For this review, take the finished solid that the model builds, in its own axes (mm). A direction names the side the tool comes from. Coordinates: 2 decimals unless noted, no trailing zeros. Loops run counter-clockwise (first coordinate to the right, second up) from the corner with the lowest first, then second, coordinate; pieces in that order, holes last. Notation, with made-up numbers: M -18.5,21.25 L 8.5,21.25 A35 cw 8.5,56.25 Z; hole C 58.5,38 d9. An arc over 180 degrees is marked long. Use one line per item in the form item = value.
```python
from build123d import *

# Parameters (mm, degrees)
SKETCH1_W           = 50
SKETCH1_H           = 50
BOSS_EXTRUDE1_DEPTH = 10
CUT_EXTRUDE3_DEPTH  = 6.3
SKETCH5_R           = 9
SKETCH5_R_2         = 3.1
BOSS_EXTRUDE2_DEPTH = 6
SKETCH6_R           = 2.7
BOSS_EXTRUDE3_DEPTH = 2.5
FILLET1_R           = 0.5
CUT_EXTRUDE4_DEPTH  = 57.789083458
FILLET2_R           = 5
CHAMFER1_SIZE       = 1
CHAMFER2_SIZE       = 1
CHAMFER2_SIZE2      = 1.414213562
FILLET3_R           = 2
SKETCH9_R           = 3.1
CUT_EXTRUDE5_DEPTH  = 37.434050008
CHAMFER3_SIZE       = 1
CUT_EXTRUDE6_DEPTH  = 6
FILLET4_R           = 3


with BuildPart() as part:
    # Sketch1 → Boss-Extrude1 (new body)
    with BuildSketch(Plane(origin=(0, 0, 0), x_dir=(1, 0, 0), z_dir=(0, 1, 0))):
        Rectangle(SKETCH1_W, SKETCH1_H)
    extrude(amount=BOSS_EXTRUDE1_DEPTH)

    # Sketch4 → Cut-Extrude3 (cut)
    with BuildSketch(Plane(origin=(0, 0, 0), x_dir=(-1, 0, 0), z_dir=(0, -1, 0))):
        with BuildLine():
            Line((21, -7.228416147), (21, -10.5))
            ThreePointArc((21, -10.5), (20.267766953, -12.267766953), (18.5, -13))
            Line((18.5, -13), (-18.5, -13))
            ThreePointArc((-18.5, -13), (-20.267766953, -12.267766953), (-21, -10.5))
            Line((-21, -10.5), (-21, -7.228416147))
            ThreePointArc((-21, -7.228416147), (-20.591644852, -6.017356006), (-19.533333333, -5.300838508))
            ThreePointArc((-19.533333333, -5.300838508), (-15.5, 0), (-19.533333333, 5.300838508))
            ThreePointArc((-19.533333333, 5.300838508), (-20.591644852, 6.017356006), (-21, 7.228416147))
            Line((-21, 7.228416147), (-21, 10.5))
            ThreePointArc((-21, 10.5), (-20.267766953, 12.267766953), (-18.5, 13))
            Line((-18.5, 13), (18.5, 13))
            ThreePointArc((18.5, 13), (20.267766953, 12.267766953), (21, 10.5))
            Line((21, 10.5), (21, 7.228416147))
            ThreePointArc((21, 7.228416147), (20.591644852, 6.017356006), (19.533333333, 5.300838508))
            ThreePointArc((19.533333333, 5.300838508), (15.5, 0), (19.533333333, -5.300838508))
            ThreePointArc((19.533333333, -5.300838508), (20.591644852, -6.017356006), (21, -7.228416147))
        make_face()
    extrude(amount=-CUT_EXTRUDE3_DEPTH, mode=Mode.SUBTRACT)

    # Sketch5 → Boss-Extrude2 (add)
    with BuildSketch(Plane(origin=(0, 6.3, 0), x_dir=(-1, 0, 0), z_dir=(0, -1, 0))):
        with Locations(Location((0, 0, 0), (0, 0, 90))):
            Circle(SKETCH5_R)
        with Locations(Location((0, 0, 0), (0, 0, 90))):
            Circle(SKETCH5_R_2, mode=Mode.SUBTRACT)
    extrude(amount=BOSS_EXTRUDE2_DEPTH)

    # Sketch6 → Boss-Extrude3 (add)
    with BuildSketch(Plane.XZ):
        with Locations(Location((-20, 0, 0), (0, 0, 90))):
            Circle(SKETCH6_R)
        with Locations(Location((20, 0, 0), (0, 0, 90))):
            Circle(SKETCH6_R)
    extrude(amount=BOSS_EXTRUDE3_DEPTH)

    # Fillet1
    fillet1_edges = [part.edges().sort_by_distance(p)[0] for p in [
        (-20, -2.5, -2.7),
        (20, -2.5, -2.7),
    ]]
    fillet(fillet1_edges, radius=FILLET1_R)

    # Sketch8 → Cut-Extrude4 (cut, through all)
    with BuildSketch(Plane(origin=(25, 0, 0), x_dir=(0, 0, -1), z_dir=(1, 0, 0))):
        Polygon((-25, 0), (-25, 5), (-15.5, 5), (-20.5, 0), align=None)
        Polygon((25, 0), (25, 5), (15.5, 5), (20.5, 0), align=None)
    extrude(amount=-CUT_EXTRUDE4_DEPTH, mode=Mode.SUBTRACT)

    # Fillet2
    fillet2_edges = [part.edges().sort_by_distance(p)[0] for p in [
        (-25, 7.5, -25),
        (25, 7.5, -25),
        (25, 7.5, 25),
        (-25, 7.5, 25),
    ]]
    fillet(fillet2_edges, radius=FILLET2_R)

    # Chamfer1
    chamfer1_edges = [part.edges().sort_by_distance(p)[0] for p in [
        (0, 10, -25),
        (25, 10, 0),
        (-25, 10, 0),
        (0, 10, 25),
        (23.535533906, 10, 23.535533906),
        (-23.535533906, 10, 23.535533906),
        (-23.535533906, 10, -23.535533906),
        (23.535533906, 10, -23.535533906),
    ]]
    chamfer(chamfer1_edges, length=CHAMFER1_SIZE)

    # Chamfer2
    chamfer2_edges = [part.edges().sort_by_distance(p)[0] for p in [
        (0, 0, 20.5),
        (0, 0, -20.5),
    ]]
    chamfer2_side = [part.faces().sort_by_distance(p)[0] for p in [
        (24.353393474, 0, 0),
    ]]
    chamfer(chamfer2_edges, length=CHAMFER2_SIZE, length2=CHAMFER2_SIZE2, reference=chamfer2_side[0])

    # Fillet3
    fillet3_edges = [part.edges().sort_by_distance(p)[0] for p in [
        (25, 0.5, -19.5),
        (25, 0.5, 19.5),
        (-25, 0.5, -19.5),
        (-25, 0.5, 19.5),
    ]]
    fillet(fillet3_edges, radius=FILLET3_R)

    # Sketch9 → Cut-Extrude5 (cut, through all)
    with BuildSketch(Plane(origin=(0, 6.3, 0), x_dir=(-1, 0, 0), z_dir=(0, -1, 0))):
        with Locations(Location((0, 0, 0), (0, 0, 90))):
            Circle(SKETCH9_R)
    extrude(amount=-CUT_EXTRUDE5_DEPTH, mode=Mode.SUBTRACT)

    # Chamfer3
    chamfer3_edges = [part.edges().sort_by_distance(p)[0] for p in [
        (0, 10, 3.1),
    ]]
    chamfer(chamfer3_edges, length=CHAMFER3_SIZE)

    # Sketch10 → Cut-Extrude6 (cut)
    with BuildSketch(Plane(origin=(0, 0.3, 0), x_dir=(-1, 0, 0), z_dir=(0, -1, 0))):
        Polygon((3.31, -5.733088173), (6.62, 0), (3.31, 5.733088173), (-3.31, 5.733088173), (-6.62, 0), (-3.31, -5.733088173), align=None)
    extrude(amount=-CUT_EXTRUDE6_DEPTH, mode=Mode.SUBTRACT)

    # Fillet4
    fillet4_edges = [part.edges().sort_by_distance(p)[0] for p in [
        (0, 6.3, 9),
    ]]
    fillet(fillet4_edges, radius=FILLET4_R)


solid = part.part
```
1. For pin 1 Ø5 at (x, z) = (-8, -18.5) entering from -Y; pin 2 Ø3.5 at (x, z) = (-2, -1.5) entering from -Y; pin 3 Ø1.1 at (x, y) = (9.5, 0.5) entering from -Z, all flat-tipped, find the tip position at first contact; note any pin that passes through.
Computed values:
pin_1 = 0
pin_2 = 6.3
pin_3 = -19.5
2. Wall thickness on line 1 along X through (y, z) = (1.75, 0); line 2 along Z through (x, y) = (2.5, 5.5); line 3 along X through (y, z) = (8.35, 0): over which ranges is each line inside the solid? List them lowest first. Write a range as from..to.
Computed values:
line_1 = -25..-15.5, -9..-6.62, 6.62..9, 15.5..25
line_2 = -25..-13, -9.64..-5.73, 5.73..9.64, 13..25
line_3 = -25..-3.1, 3.1..25
3. Draft analysis for pull direction X (two halves, no side actions). For faces 1 (the face through (21, 3, -9)), 2 (the face through (-4.94, 3.26, 2.91)), 3 (the face through (22.996, 9.715, -23.063)), 4 (the face through (0.3, 3, -17.5)), state which applies: +X half, -X half, draft (parallel to the pull), parting line (faces both ways), or undercut.
Computed values:
face_1 = undercut
face_2 = undercut
face_3 = +X half
face_4 = draft
4. Tool access review of faces 5 (the face through (0, 5, -20)), 6 (the face through (17.323, -0.986, -0.351)), 7 (the face through (0.3, 3, 17.5)), 8 (the face through (0, 10, -6)): name each direction out of +Z, -Z, +X, -X, +Y, -Y from which nothing blocks a thin tool from reaching the whole face with its end or side.
Computed values:
face_5 = -Z, +X, -X
face_6 = -Y
face_7 = +Z, +X, -X
face_8 = +Z, -Z, +X, -X, +Y
5. Consider section B-B on y = 4. Write out the cut boundary in (x, z).
Computed values:
outline = M -25,-16.5 L 25,-16.5 L 25,16.5 L -25,16.5 Z; C 0,0 d18.17; hole M -21,-10.5 A2.5 ccw -18.5,-13 L 18.5,-13 A2.5 ccw 21,-10.5 L 21,-7.23 A2 ccw 19.53,-5.3 A5.5 cw 19.53,5.3 A2 ccw 21,7.23 L 21,10.5 A2.5 ccw 18.5,13 L -18.5,13 A2.5 ccw -21,10.5 L -21,7.23 A2 ccw -19.53,5.3 A5.5 cw -19.53,-5.3 A2 ccw -21,-7.23 Z; hole M -6.62,0 L -3.31,-5.73 L 3.31,-5.73 L 6.62,0 L 3.31,5.73 L -3.31,5.73 Z
6. Consider section C-C on x = 14. Write out the cut boundary in (y, z).
Computed values:
outline = M 0,-19.5 L 1,-19.5 L 5,-15.5 L 5,-25 L 9,-25 L 10,-24 L 10,24 L 9,25 L 5,25 L 5,15.5 L 1,19.5 L 0,19.5 L 0,13 L 6.3,13 L 6.3,-13 L 0,-13 Z
